The listing builds one solid part. Answer for the finished solid, in the listing's coordinates (mm). Give positions to 0.01 mm unless a question says otherwise; leave off trailing zeros. Order: outer loops, then holes, each group sorted by start corner. A loop starts at its lowest first (then second) coordinate and runs counter-clockwise, first axis right, second up. Notation, with made-up numbers: (72, 61) - (102, 61) arc R9 cw to (102, 67) - close; hole circle Ø10 at (79, 68). An arc over 180 degrees is marked (long way). Use a Markdown table: item, result. Add a question column.
1) Find section C-C, the plane y = -6.25. State how many separate pieces and enclosed holes the cut face has, plus the area to 3 significant figures.
2) Find section B-B, the plane x = 25. Determine the outline of the cut face in (y, z).
3) Find section A-A, the plane z = -1.5. Determine the outline of the cut face in (x, y).
4) Straight lines are drawn through the part: line 1 (Z direction, x = 1.5, y = -7.5); line 2 (X direction, y = -4.5, z = 3.5); line 3 (X direction, y = -8.25, z = -0.75). For each, find the intervals that lie inside material, in ascending order.
5) Flat-ended cylindrical pins translate along their axes: pin 1 (1 mm diameter, centred on x = 12, y = -8.5, fed in from -Z); pin 2 (2.5 mm diameter, centred on x = 24.69, z = 2.57, fed in from -Y); pin 3 (1.5 mm diameter, centred on x = 11.5, y = -9, fed in from +Z); pin 4 (1 mm diameter, centred on y = -7, z = 5.5, fed in from -X). Find the tip coordinate at first contact, or state that the pin passes through.
6) Find section D-D, the plane x = 8. Determine the outline of the cut face in (y, z), plus the area to 3 significant figures.
7) The mould has two halves that part along X. Classify faces 1 (the face through (26.076, -7.148, 1.997)), 2 (the face through (16, -7, 0)), 3 (the face through (-0.07, -7.148, -3.174)): released by +X, released by -X, zero draft, split by the parting line, or undercut.
from build123d import *

# Parameters (mm, degrees)
F0_R     = 1.5
F1_DEPTH = 14.5
F0_R_2   = 2
F2_DEPTH = 14.5


with BuildPart() as f1:
    # F0 (on Front) → F1 (new body)
    with BuildSketch(Plane.XZ):
        with BuildLine():
            ThreePointArc((-2.9066747097, 1.2774455495), (0.6526610133, 3.1071946514), (3.175, 0))
            Line((3.175, 0), (29, 0))
            ThreePointArc((29, 0), (13.5651610133, 13.5892229178), (-2.9066747097, 1.2774455495))
        make_face()
        with Locations((24.690752849, 2.5710954797)):
            Circle(F0_R, mode=Mode.SUBTRACT)
    extrude(amount=F1_DEPTH)

    # F0 (on Front) → F2 (join)
    with BuildSketch(Plane.XZ):
        with BuildLine():
            ThreePointArc((-2.9066747097, 1.2774455495), (0.6526610133, 3.1071946514), (3.175, 0))
            Line((3.175, 0), (29, 0))
            ThreePointArc((29, 0), (13.5651610133, 13.5892229178), (-2.9066747097, 1.2774455495))
        make_face()
        with Locations((24.690752849, 2.5710954797)):
            Circle(F0_R, mode=Mode.SUBTRACT)
        with BuildLine():
            ThreePointArc((-3.175, 0), (0, -3.175), (3.175, 0))
            ThreePointArc((3.175, 0), (0.6526610133, 3.1071946514), (-2.9066747097, 1.2774455495))
            ThreePointArc((-2.9066747097, 1.2774455495), (-3.053618487, 0.6414074301), (-3.175, 0))
        make_face()
        Circle(F0_R_2, mode=Mode.SUBTRACT)
    extrude(amount=F2_DEPTH)


solid = f1.part
The answers:
| question | item | result |
|---|---|---|
| 1 | separate pieces | 1 |
| 1 | enclosed holes | 2 |
| 1 | area | 326 mm2 |
| 2 | outline | (-14.5, 0) - (0, 0) - (0, 1.1) - (-14.5, 1.1) - close; (-14.5, 4.04) - (0, 4.04) - (0, 8.24) - (-14.5, 8.24) - close |
| 3 | outline | (-2.8, -14.5) - (-1.32, -14.5) - (-1.32, 0) - (-2.8, 0) - close; (1.32, -14.5) - (2.8, -14.5) - (2.8, 0) - (1.32, 0) - close |
| 4 | line 1 | -2.8 to -1.32, 1.32 to 8.95 |
| 4 | line 2 | -2.17 to 23.51, 25.87 to 28 |
| 4 | line 3 | -3.09 to -1.85, 1.85 to 3.09 |
| 5 | pin 1 | z = 0 |
| 5 | pin 2 | through |
| 5 | pin 3 | z = 13.59 |
| 5 | pin 4 | x = -1.46 |
| 6 | outline | (-14.5, 0) - (0, 0) - (0, 12.85) - (-14.5, 12.85) - close |
| 6 | area | 186 mm2 |
| 7 | face 1 | undercut |
| 7 | face 2 | zero draft |
| 7 | face 3 | split by the parting line |
